Check sheet for the modelled part. Datum: model origin and axes. Units: mm. A direction names the side the tool comes from. Give positions to 0.01 mm unless a question says otherwise; leave off trailing zeros. Order: outer loops, then holes, each group sorted by start corner. A loop starts at its lowest first (then second) coordinate and runs counter-clockwise, first axis right, second up. Notation, with made-up numbers: (24, -31) -> (72, -31) arc R23 cw to (72, -12) -> close; hole circle Ø11 at (14, -37.75). An arc over 180 degrees is marked (long way). Answer in a Markdown table with one row per item. Add a question column.
(1) Thickness scan on L1, parallel to X at y = 4.25, z = 137; L2, parallel to X at y = 4.75, z = 131.5; L3, parallel to Z at x = -43.5, y = 5.5. Record the ranges inside material, lowest first. Write a range as [from, to].
(2) Cross-section at B-B (x = -91). Record the cut outline in (y, z), then the cut area to 3 significant figures.
(3) Set-up check for faces 4 (the face through (-13, 4, 109.959)), 5 (the face through (-20.316, 3.574, 129.299)), 6 (the face through (-110, 4, 6.583)): record each of +Z, -Z, +X, -X, +Y, -Y from which the full face is reachable in a straight line by a thin tool's end or side.
(4) Cross-section at A-A (z = 58). Record the cut outline in (x, y), then the cut area to 3 significant figures.
(5) Release check for a two-part mould opening along Z. For faces 1 (the face through (-26, 6.25, 139)), 2 (the face through (-21.262, 3.574, 119.648)), 3 (the face through (-16.418, 3.574, 114.493)) record: released by +Z, released by -Z, zero draft, split by the parting line, or undercut.
(6) Go/stop test with flat-tipped pins: pin 1 (1.3 mm diameter, centred on x = -29, z = 141.01, fed in from +Y); pin 2 (1 mm diameter, centred on x = -51, y = 4.5, fed in from -Z); pin 3 (7 mm diameter, centred on x = -28, z = 137.5, fed in from +Y); pin 4 (3 mm diameter, centred on y = 3.5, z = 137.5, fed in from -X). Record where each tip stops, or that it passes through.
```python
from build123d import *

# Parameters (mm, degrees)
BOSS_EXTRUDE1_DEPTH = 7.25
CUT_EXTRUDE2_DEPTH  = 2
SKETCH6_R           = 1.05
CUT_EXTRUDE3_DEPTH  = 184.988971882
FILLET1_R           = 1
CUT_EXTRUDE6_DEPTH  = 10
SKETCH14_R          = 1.05
CUT_EXTRUDE7_DEPTH  = 5
FILLET3_R           = 1
FILLET4_R           = 10
SKETCH16_W          = 40
SKETCH16_H          = 15
CUT_EXTRUDE8_DEPTH  = 1
FILLET5_R           = 2


with BuildPart() as part:
    # Sketch2 → Boss-Extrude1 (new body)
    with BuildSketch(Plane(origin=(0, 0, 0), x_dir=(1, 0, 0), z_dir=(0, 1, 0))):
        with BuildLine():
            Line((-17.623152329, -113.641649504), (-22.623152329, -118.641649504))
            ThreePointArc((-22.623152329, -118.641649504), (-20.659920019, -126.747167143), (-20, -135.060902938))
            Line((-20, -135.060902938), (-20, -143.510902938))
            Line((-20, -143.510902938), (-32, -143.510902938))
            Line((-32, -143.510902938), (-32, -135.060902938))
            ThreePointArc((-32, -135.060902938), (-35.097995018, -119.486230235), (-43.920338415, -106.282660267))
            ThreePointArc((-43.920338415, -106.282660267), (-94.299467161, -65.822568266), (-114.908659431, -4.582574373))
            Line((-114.908659431, -4.582574373), (-104.899952393, -4.582574373))
            ThreePointArc((-104.899952393, -4.582574373), (-73.684211281, -74.803990588), (-3, -104.957134107))
            Line((-3, -104.957134107), (-3, -114.960862906))
            ThreePointArc((-3, -114.960862906), (-10.332651354, -114.534869433), (-17.623152329, -113.641649504))
        make_face()
    extrude(amount=BOSS_EXTRUDE1_DEPTH)

    # Sketch4 → Cut-Extrude2 (cut)
    with BuildSketch(Plane(origin=(0, 0, 4.582574373), x_dir=(-1, 0, 0), z_dir=(0, 0, -1))):
        Polygon((111.556991832, 5.27912492), (109.29813467, 5.883330451), (107.64544875, 4.229205531), (108.251619992, 1.97087508), (110.510477153, 1.366669549), (112.163163073, 3.020794469), align=None)
    extrude(amount=-CUT_EXTRUDE2_DEPTH, mode=Mode.SUBTRACT)

    # Sketch6 → Cut-Extrude3 (cut, through all)
    with BuildSketch(Plane(origin=(0, 7.25, 0), x_dir=(1, 0, 0), z_dir=(0, 1, 0))):
        with Locations(Location((-29, -141.010902938, 0), (0, 0, 270))):
            Circle(SKETCH6_R)
        with Locations(Location((-23, -141.010902938, 0), (0, 0, 270))):
            Circle(SKETCH6_R)
    extrude(amount=-CUT_EXTRUDE3_DEPTH, mode=Mode.SUBTRACT)

    # Fillet1
    fillet1_edges = [part.edges().sort_by_distance(p)[0] for p in [
        (-26, 0, 143.510902938),
        (-20, 3.625, 143.510902938),
        (-32, 3.625, 143.510902938),
        (-26, 7.25, 143.510902938),
    ]]
    fillet(fillet1_edges, radius=FILLET1_R)

    # Sketch13 → Cut-Extrude6 (cut)
    with BuildSketch(Plane(origin=(0, 7.25, 0), x_dir=(1, 0, 0), z_dir=(0, 1, 0))):
        with BuildLine():
            Line((-8, -109.958998506), (-19, -109.958998506))
            ThreePointArc((-19, -109.958998506), (-30.884750495, -107.29264995), (-40.491380382, -99.804701556))
            ThreePointArc((-40.491380382, -99.804701556), (-44.399963721, -95.911179829), (-49, -92.86549413))
            Line((-49, -92.86549413), (-8, -92.86549413))
            Line((-8, -92.86549413), (-8, -109.958998506))
        make_face()
    extrude(amount=-CUT_EXTRUDE6_DEPTH, mode=Mode.SUBTRACT)

    # Sketch14 → Cut-Extrude7 (cut)
    with BuildSketch(Plane(origin=(-3, 0, 0), x_dir=(0, 0, -1), z_dir=(1, 0, 0))):
        with Locations((-107.458066307, 3.625)):
            Circle(SKETCH14_R)
    extrude(amount=-CUT_EXTRUDE7_DEPTH, mode=Mode.SUBTRACT)

    # Fillet3
    fillet3_edges = [part.edges().sort_by_distance(p)[0] for p in [
        (-8, 3.625, 104.694794522),
    ]]
    fillet(fillet3_edges, radius=FILLET3_R)

    # Fillet4
    # the kernel refuses this fillet: 10 mm, written as the material it adds along each edge
    with BuildSketch(Plane(origin=(-22.623152329, 0, 118.641649504), x_dir=(0.7071067811865469, 0, -0.7071067811865481), z_dir=(0, 1, 0))) as fillet4_piece_1:
        with BuildLine():
            CenterArc((5.789991957, -10), FILLET4_R, 90, 57.380097375)
            ThreePointArc((-2.632659996, -4.609366079), (-1.258256696, -2.337851865), (0, 0))
            Line((0, 0), (5.789991957, 0))
        make_face()
    extrude(amount=7.25)
    with BuildSketch(Plane(origin=(-17.623152329, 0, 113.641649504), x_dir=(0.9911373960250678, 0, 0.13284073998833376), z_dir=(0, 1, 0))) as fillet4_piece_2:
        with BuildLine():
            CenterArc((4.947598948, -9.997874884), FILLET4_R, 91.18123592, 51.452542901)
            Line((-3.000126671, -3.928801026), (0, 0))
            ThreePointArc((0, 0), (2.370724496, -0.024438834), (4.741448992, 0))
        make_face()
    extrude(amount=7.25)

    # Sketch16 → Cut-Extrude8 (cut)
    with BuildSketch(Plane(origin=(0, 7.25, 0), x_dir=(1, 0, 0), z_dir=(0, 1, 0))):
        with Locations((-25.357096051, -142.5)):
            Rectangle(SKETCH16_W, SKETCH16_H)
    extrude(amount=-CUT_EXTRUDE8_DEPTH, mode=Mode.SUBTRACT)

    # Fillet5
    # the kernel refuses this fillet: 2 mm, written as the material it takes off along each edge
    with BuildSketch(Plane(origin=(-15.669908173, 7.25, 135), x_dir=(0, 0, -1), z_dir=(-1, 0, 0))) as fillet5_piece_1:
        with BuildLine():
            CenterArc((1.732050808, 2), FILLET5_R, 210, 60)
            Line((0, 1), (-0.034641016, 0.98))
            ThreePointArc((-0.034641016, 0.98), (-0.04, 0.5), (-0.04, 0))
            Line((-0.04, 0), (0, -0.04))
            Line((0, -0.04), (1.732050808, -0.04))
            Line((1.732050808, -0.04), (1.732050808, 0))
        make_face()
    extrude(amount=20.660264414, mode=Mode.SUBTRACT)


solid = part.part
```
Answer below:
| question | item | result |
|---|---|---|
| 1 | L1 | x = [-32, -20] |
| 1 | L2 | x = [-32.16, -20.12] |
| 1 | L3 | z = [96.68, 106.71] |
| 2 | outline | (0, 52.38) -> (7.25, 52.38) -> (7.25, 70.31) -> (0, 70.31) -> close |
| 2 | area | 130 mm² |
| 3 | face 4 | -Z, +Y, -Y |
| 3 | face 5 | +X, +Y, -Y |
| 3 | face 6 | -Z |
| 4 | outline | (-99.3, 0) -> (-87.53, 0) -> (-87.53, 7.25) -> (-99.3, 7.25) -> close |
| 4 | area | 85.4 mm² |
| 5 | face 1 | zero draft |
| 5 | face 2 | undercut |
| 5 | face 3 | released by +Z |
| 6 | pin 1 | passes through |
| 6 | pin 2 | stops at z = 91.5 |
| 6 | pin 3 | stops at y = 7.11 |
| 6 | pin 4 | stops at x = -32 |
